from build123d import *

# Parameters (mm, degrees)
CROQUIS1_W                   = 30
CROQUIS1_H                   = 20
SALIENTE_EXTRUIR1_DEPTH      = 5
SALIENTE_EXTRUIR2_DEPTH      = 3
SALIENTE_EXTRUIR2_DEPTH_BACK = 3
CROQUIS4_R                   = 2.1
CORTAR_EXTRUIR1_DEPTH        = 7


with BuildPart() as part:
    # Croquis1 → Saliente-Extruir1 (new body)
    with BuildSketch(Plane.XY):
        Rectangle(CROQUIS1_W, CROQUIS1_H)
    extrude(amount=SALIENTE_EXTRUIR1_DEPTH)

    # Croquis3 → Saliente-Extruir2 (add, two sides)
    with BuildSketch(Plane(origin=(0, 0, 0), x_dir=(1, 0, 0), z_dir=(0, 1, 0))) as saliente_extruir2_sk:
        Polygon((-4, 0), (4, 0), (9.142300877, 6.128355545), (4.546034219, 9.985081203), align=None)
    extrude(amount=SALIENTE_EXTRUIR2_DEPTH)
    extrude(saliente_extruir2_sk.sketch, amount=-SALIENTE_EXTRUIR2_DEPTH_BACK)

    # Croquis4 → Cortar-Extruir1 (cut)
    with BuildSketch(Plane(origin=(6.795004522, 0, -8.097971051), x_dir=(-0.766044443, 0, -0.64278761), z_dir=(0.64278761, 0, -0.766044443))):
        Circle(CROQUIS4_R)
    extrude(amount=-CORTAR_EXTRUIR1_DEPTH, mode=Mode.SUBTRACT)


solid = part.part
CAD build for the part. Positions are in the model's coordinates, mm. A direction names the side the tool comes from. Give positions to 0.01 mm unless a question says otherwise; leave off trailing zeros. Order: outer loops, then holes, each group sorted by start corner. A loop starts at its lowest first (then second) coordinate and runs counter-clockwise, first axis right, second up. Notation, with made-up numbers: (36, 79.25) -> (94, 79.25) arc R19 cw to (94, 114.25) -> close; hole circle Ø5 at (-29, -0.5). An arc over 180 degrees is marked (long way). Return JSON: item names as keys, results as strings.
Q1. Drill centre lines: line 1 (Z direction, x = -4, y = -8.75); line 2 (Y direction, x = 3.75, z = -6.75); line 3 (Y direction, x = 4.5, z = -7.25). Where is each one in solid material? Low to high.
Working result:
{"line 1": "0 to 5", "line 2": "-3 to -1.5, 1.5 to 3", "line 3": "-3 to -1.71, 1.71 to 3"}
Q2. Saw through at C-C (x = 11.75). Write the cut outline in (y, z).
Working result:
{"outline": "(-10, 0) -> (10, 0) -> (10, 5) -> (-10, 5) -> close"}
Q3. Which spindle directions (+Z, -Z, +X, -X, +Y, -Y) get a long thin tool onto all of the face, cutting with end or side? Do faces 5 (the face through (-15, 0, 2)), 6 (the face through (2, 3, -4)), 7 (the face through (6.535, 0.042, -3.021)). Say none if no direction does.
Working result:
{"face 5": "+Z, -Z, -X, +Y, -Y", "face 6": "-Z, +X, -X, +Y", "face 7": "+X, +Y, -Y"}
Q4. Mould opens along Z. For faces 1 (the face through (0, 0, 5)), 2 (the face through (2.318, 0.029, -2.717)), 3 (the face through (2, -3, -4)), 4 (the face through (6.184, 0.092, -4.106)) say: pulls with the +Z half, pulls with the -Z half, needs draft (parallel to the pull), parting line crosses it, or undercut.
Working result:
{"face 1": "pulls with the +Z half", "face 2": "undercut", "face 3": "needs draft", "face 4": "undercut"}
Q5. Saw through at B-B (y = -1.75). Write the cut outline in (x, z), then the cut area to 3 significant figures.
Working result:
{"outline": "(-15, 0) -> (-4, 0) -> (4.55, -9.99) -> (5.91, -8.84) -> (1.41, -3.48) -> (3.18, -1.99) -> (7.68, -7.35) -> (9.14, -6.13) -> (4, 0) -> (15, 0) -> (15, 5) -> (-15, 5) -> close", "area": "198 mm²"}
Q6. Flat gauge pins, fed straight in: pin 1 (6 mm diameter, centred on x = -2.5, y = 2.5, fed in from -Z); pin 2 (1.5 mm diameter, centred on x = 3.5, y = 1, fed in from -Z); pin 3 (2 mm diameter, centred on x = 3, y = -6, fed in from -Z). Where does each tip first touch, or does it go through?
Working result:
{"pin 1": "z = -5.26", "pin 2": "z = -9.64", "pin 3": "z = 0"}
Q7. Saw through at D-D (y = -4.75). Write the cut outline in (x, z).
Working result:
{"outline": "(-15, 0) -> (15, 0) -> (15, 5) -> (-15, 5) -> close"}
Q8. Saw through at A-A (x = -0.5). Write the cut outline in (y, z).
Working result:
{"outline": "(-10, 0) -> (-3, 0) -> (-3, -4.09) -> (3, -4.09) -> (3, 0) -> (10, 0) -> (10, 5) -> (-10, 5) -> close"}
